Check sheet for the modelled part. Datum: model origin and axes. Units: mm. Face numbers are marked on the shaded views. Round coordinates to 2 decimals unless told otherwise and drop trailing zeros. Order: outer loops, then holes, each group sorted by start corner. A loop starts at its lowest first (then second) coordinate and runs counter-clockwise, first axis right, second up. Notation, with made-up numbers: (14.25, 16.5) -> (32.25, 16.5) arc R27 cw to (32.25, 49.5) -> close; hole circle Ø11 at (-30.5, 70). An arc over 180 degrees is marked (long way). Answer in a Markdown table with one row per item.
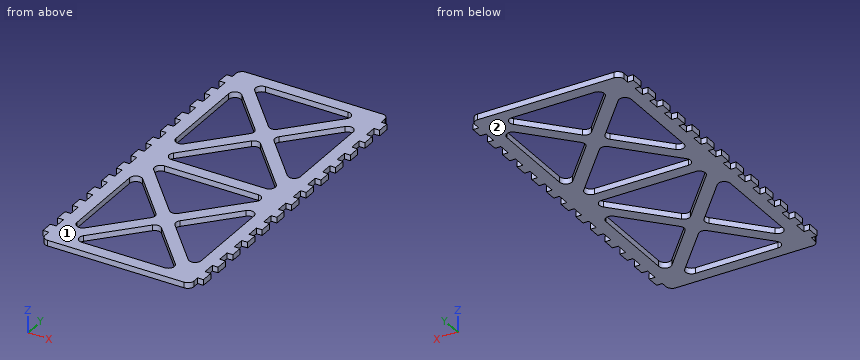
from build123d import *

# Parameters (mm, degrees)
SKETCH1_W                = 77.47
SKETCH1_H                = 171.45
BOSS_EXTRUDE1_DEPTH      = 1.4605
SKETCH3_W                = 2.921
SKETCH3_H                = 6.35
BOSS_EXTRUDE2_DEPTH      = 3
LPATTERN1_COUNT          = 13
LPATTERN1_PITCH          = 12.7
MIRROR1_COPY_1_SKETCH_W  = 2.921
MIRROR1_COPY_1_SKETCH_H  = 6.35
MIRROR1_COPY_1_DEPTH     = 3
MIRROR1_COPY_2_SKETCH_W  = 2.921
MIRROR1_COPY_2_SKETCH_H  = 6.35
MIRROR1_COPY_2_DEPTH     = 3
MIRROR1_COPY_3_SKETCH_W  = 2.921
MIRROR1_COPY_3_SKETCH_H  = 6.35
MIRROR1_COPY_3_DEPTH     = 3
MIRROR1_COPY_4_SKETCH_W  = 2.921
MIRROR1_COPY_4_SKETCH_H  = 6.35
MIRROR1_COPY_4_DEPTH     = 3
MIRROR1_COPY_5_SKETCH_W  = 2.921
MIRROR1_COPY_5_SKETCH_H  = 6.35
MIRROR1_COPY_5_DEPTH     = 3
MIRROR1_COPY_6_SKETCH_W  = 2.921
MIRROR1_COPY_6_SKETCH_H  = 6.35
MIRROR1_COPY_6_DEPTH     = 3
MIRROR1_COPY_7_SKETCH_W  = 2.921
MIRROR1_COPY_7_SKETCH_H  = 6.35
MIRROR1_COPY_7_DEPTH     = 3
MIRROR1_COPY_8_SKETCH_W  = 2.921
MIRROR1_COPY_8_SKETCH_H  = 6.35
MIRROR1_COPY_8_DEPTH     = 3
MIRROR1_COPY_9_SKETCH_W  = 2.921
MIRROR1_COPY_9_SKETCH_H  = 6.35
MIRROR1_COPY_9_DEPTH     = 3
MIRROR1_COPY_10_SKETCH_W = 2.921
MIRROR1_COPY_10_SKETCH_H = 6.35
MIRROR1_COPY_10_DEPTH    = 3
MIRROR1_COPY_11_SKETCH_W = 2.921
MIRROR1_COPY_11_SKETCH_H = 6.35
MIRROR1_COPY_11_DEPTH    = 3
MIRROR1_COPY_12_SKETCH_W = 2.921
MIRROR1_COPY_12_SKETCH_H = 6.35
MIRROR1_COPY_12_DEPTH    = 3
CUT_EXTRUDE1_DEPTH       = 96.389297571
FILLET1_R                = 3.175
FILLET2_R                = 3.175


with BuildPart() as part:
    # Sketch1 → Boss-Extrude1 (new, symmetric)
    with BuildSketch(Plane.XY):
        Rectangle(SKETCH1_W, SKETCH1_H)
    extrude(amount=BOSS_EXTRUDE1_DEPTH, both=True)

    # Sketch3 → Boss-Extrude2 (add)
    with BuildSketch(Plane.ZY.offset(38.735)):
        with Locations((0, -76.2)):
            Rectangle(SKETCH3_W, SKETCH3_H)
    boss_extrude2 = extrude(amount=BOSS_EXTRUDE2_DEPTH)

    # LPattern1: Boss-Extrude2 ×13
    with Locations(*[(0, i * LPATTERN1_PITCH, 0) for i in range(1, LPATTERN1_COUNT)]):
        add(boss_extrude2)

    # Mirror1: Boss-Extrude2 across plane
    add(boss_extrude2.mirror(Plane.ZY))

    # Mirror1 copy 1 sketch → Mirror1 copy 1 (add)
    with BuildSketch(Plane(origin=(38.735, 12.7, 0), x_dir=(0, 0, 1), z_dir=(1, 0, 0))):
        with Locations((0, 76.2)):
            Rectangle(MIRROR1_COPY_1_SKETCH_W, MIRROR1_COPY_1_SKETCH_H)
    extrude(amount=MIRROR1_COPY_1_DEPTH)

    # Mirror1 copy 2 sketch → Mirror1 copy 2 (add)
    with BuildSketch(Plane(origin=(38.735, 25.4, 0), x_dir=(0, 0, 1), z_dir=(1, 0, 0))):
        with Locations((0, 76.2)):
            Rectangle(MIRROR1_COPY_2_SKETCH_W, MIRROR1_COPY_2_SKETCH_H)
    extrude(amount=MIRROR1_COPY_2_DEPTH)

    # Mirror1 copy 3 sketch → Mirror1 copy 3 (add)
    with BuildSketch(Plane(origin=(38.735, 38.1, 0), x_dir=(0, 0, 1), z_dir=(1, 0, 0))):
        with Locations((0, 76.2)):
            Rectangle(MIRROR1_COPY_3_SKETCH_W, MIRROR1_COPY_3_SKETCH_H)
    extrude(amount=MIRROR1_COPY_3_DEPTH)

    # Mirror1 copy 4 sketch → Mirror1 copy 4 (add)
    with BuildSketch(Plane(origin=(38.735, 50.8, 0), x_dir=(0, 0, 1), z_dir=(1, 0, 0))):
        with Locations((0, 76.2)):
            Rectangle(MIRROR1_COPY_4_SKETCH_W, MIRROR1_COPY_4_SKETCH_H)
    extrude(amount=MIRROR1_COPY_4_DEPTH)

    # Mirror1 copy 5 sketch → Mirror1 copy 5 (add)
    with BuildSketch(Plane(origin=(38.735, 63.5, 0), x_dir=(0, 0, 1), z_dir=(1, 0, 0))):
        with Locations((0, 76.2)):
            Rectangle(MIRROR1_COPY_5_SKETCH_W, MIRROR1_COPY_5_SKETCH_H)
    extrude(amount=MIRROR1_COPY_5_DEPTH)

    # Mirror1 copy 6 sketch → Mirror1 copy 6 (add)
    with BuildSketch(Plane(origin=(38.735, 76.2, 0), x_dir=(0, 0, 1), z_dir=(1, 0, 0))):
        with Locations((0, 76.2)):
            Rectangle(MIRROR1_COPY_6_SKETCH_W, MIRROR1_COPY_6_SKETCH_H)
    extrude(amount=MIRROR1_COPY_6_DEPTH)

    # Mirror1 copy 7 sketch → Mirror1 copy 7 (add)
    with BuildSketch(Plane(origin=(38.735, 88.9, 0), x_dir=(0, 0, 1), z_dir=(1, 0, 0))):
        with Locations((0, 76.2)):
            Rectangle(MIRROR1_COPY_7_SKETCH_W, MIRROR1_COPY_7_SKETCH_H)
    extrude(amount=MIRROR1_COPY_7_DEPTH)

    # Mirror1 copy 8 sketch → Mirror1 copy 8 (add)
    with BuildSketch(Plane(origin=(38.735, 101.6, 0), x_dir=(0, 0, 1), z_dir=(1, 0, 0))):
        with Locations((0, 76.2)):
            Rectangle(MIRROR1_COPY_8_SKETCH_W, MIRROR1_COPY_8_SKETCH_H)
    extrude(amount=MIRROR1_COPY_8_DEPTH)

    # Mirror1 copy 9 sketch → Mirror1 copy 9 (add)
    with BuildSketch(Plane(origin=(38.735, 114.3, 0), x_dir=(0, 0, 1), z_dir=(1, 0, 0))):
        with Locations((0, 76.2)):
            Rectangle(MIRROR1_COPY_9_SKETCH_W, MIRROR1_COPY_9_SKETCH_H)
    extrude(amount=MIRROR1_COPY_9_DEPTH)

    # Mirror1 copy 10 sketch → Mirror1 copy 10 (add)
    with BuildSketch(Plane(origin=(38.735, 127, 0), x_dir=(0, 0, 1), z_dir=(1, 0, 0))):
        with Locations((0, 76.2)):
            Rectangle(MIRROR1_COPY_10_SKETCH_W, MIRROR1_COPY_10_SKETCH_H)
    extrude(amount=MIRROR1_COPY_10_DEPTH)

    # Mirror1 copy 11 sketch → Mirror1 copy 11 (add)
    with BuildSketch(Plane(origin=(38.735, 139.7, 0), x_dir=(0, 0, 1), z_dir=(1, 0, 0))):
        with Locations((0, 76.2)):
            Rectangle(MIRROR1_COPY_11_SKETCH_W, MIRROR1_COPY_11_SKETCH_H)
    extrude(amount=MIRROR1_COPY_11_DEPTH)

    # Mirror1 copy 12 sketch → Mirror1 copy 12 (add)
    with BuildSketch(Plane(origin=(38.735, 152.4, 0), x_dir=(0, 0, 1), z_dir=(1, 0, 0))):
        with Locations((0, 76.2)):
            Rectangle(MIRROR1_COPY_12_SKETCH_W, MIRROR1_COPY_12_SKETCH_H)
    extrude(amount=MIRROR1_COPY_12_DEPTH)

    # Sketch4 → Cut-Extrude1 (cut, through all)
    with BuildSketch(Plane.XY.offset(1.4605)):
        Polygon((0, 47.597902846), (28.717080391, 79.375), (-28.717080391, 79.375), align=None)
        Polygon((-32.385, 11.762042191), (-4.279401091, 42.8625), (-32.385, 73.962957809), align=None)
        Polygon((32.385, 73.962957809), (4.279401091, 42.8625), (32.385, 11.762042191), align=None)
        Polygon((31.58633965, 3.175), (0, 38.127097154), (-31.58633965, 3.175), align=None)
        Polygon((-31.58633965, -3.175), (0, -38.127097154), (31.58633965, -3.175), align=None)
        Polygon((-4.279401091, -42.8625), (-32.385, -11.762042191), (-32.385, -73.962957809), align=None)
        Polygon((28.717080391, -79.375), (0, -47.597902846), (-28.717080391, -79.375), align=None)
        Polygon((32.385, -73.962957809), (32.385, -11.762042191), (4.279401091, -42.8625), align=None)
    extrude(amount=-CUT_EXTRUDE1_DEPTH, mode=Mode.SUBTRACT)

    # Fillet1
    fillet1_edges = [part.edges().sort_by_distance(p)[0] for p in [
        (-31.58633965, -3.175, 0),
        (31.58633965, -3.175, 0),
        (0, -38.127097154, 0),
        (-31.58633965, 3.175, 0),
        (0, 38.127097154, 0),
        (31.58633965, 3.175, 0),
        (32.385, 73.962957809, 0),
        (32.385, 11.762042191, 0),
        (4.279401091, 42.8625, 0),
        (-32.385, 73.962957809, 0),
        (-4.279401091, 42.8625, 0),
        (-32.385, 11.762042191, 0),
        (32.385, -11.762042191, 0),
        (32.385, -73.962957809, 0),
        (4.279401091, -42.8625, 0),
        (-32.385, -11.762042191, 0),
        (-4.279401091, -42.8625, 0),
        (-32.385, -73.962957809, 0),
        (-28.717080391, -79.375, 0),
        (0, -47.597902846, 0),
        (28.717080391, -79.375, 0),
        (-28.717080391, 79.375, 0),
        (28.717080391, 79.375, 0),
        (0, 47.597902846, 0),
    ]]
    fillet(fillet1_edges, radius=FILLET1_R)

    # Fillet2
    fillet2_edges = [part.edges().sort_by_distance(p)[0] for p in [
        (-38.735, 85.725, 0),
        (38.735, 85.725, 0),
        (38.735, -85.725, 0),
        (-38.735, -85.725, 0),
    ]]
    fillet(fillet2_edges, radius=FILLET2_R)


solid = part.part
Item 1: Cross-section at D-D (z = 0.85). State how many separate pieces and enclosed holes the cut face has, and give its area (3 significant figures).
Result sheet:
| item | result |
|---|---|
| separate pieces | 1 |
| enclosed holes | 8 |
| area | 6,460 mm^2 |
Item 2: Cross-section at A-A (y = 13.5). Record the boundary of the cut face in (x, z) (1 decimal), and give its area (3 significant figures).
Result sheet:
| item | result |
|---|---|
| outline | (-41.7, -1.5) -> (-22.3, -1.5) -> (-22.3, 1.5) -> (-41.7, 1.5) -> close; (22.3, -1.5) -> (41.7, -1.5) -> (41.7, 1.5) -> (22.3, 1.5) -> close |
| area | 114 mm^2 |
Item 3: Depth check by flat-ended pin: P1, Ø0.9, axis at x = -40.5, z = 0, coming from the -Y side (3 decimals). Enter the tip coordinate at first touch or a pass-through.
Result sheet:
| item | result |
|---|---|
| P1 | stops at y = -79.375 |
Item 4: Scan lines: line 1 (X direction, y = -42.5, z = 0.8) (3 decimals); line 2 (Y direction, x = -25.5, z = 1.2) (3 decimals); line 3 (Y direction, x = -26, z = -0.35) (3 decimals). Record each from-to range of solid material in increasing order. Write a range as [from, to].
Result sheet:
| item | result |
|---|---|
| line 1 | x = [-38.735, -32.385], [-5.405, 5.405], [32.385, 38.735] |
| line 2 | y = [-85.725, -66.344], [-19.381, -9.91], [-3.358, 3.358], [9.91, 19.381], [66.344, 85.725] |
| line 3 | y = [-85.725, -66.898], [-18.827, -9.357], [-3.586, 3.586], [9.357, 18.827], [66.898, 85.725] |
Item 5: Cross-section at C-C (y = -24). Record the boundary of the cut face in (x, z) (1 decimal), and give its area (3 significant figures).
Result sheet:
| item | result |
|---|---|
| outline | (-41.7, -1.5) -> (-32.4, -1.5) -> (-32.4, 1.5) -> (-41.7, 1.5) -> close; (-21.3, -1.5) -> (-12.8, -1.5) -> (-12.8, 1.5) -> (-21.3, 1.5) -> close; (12.8, -1.5) -> (21.3, -1.5) -> (21.3, 1.5) -> (12.8, 1.5) -> close; (32.4, -1.5) -> (41.7, -1.5) -> (41.7, 1.5) -> (32.4, 1.5) -> close |
| area | 105 mm^2 |
Item 6: Mould release check, pull along Z, two halves, no side actions. Record for the marked faces 1 and 2: pulls with the +Z half, pulls with the -Z half, needs draft (parallel to the pull), parting line crosses it, or undercut.
Result sheet:
| item | result |
|---|---|
| face 1 | pulls with the +Z half |
| face 2 | pulls with the -Z half |
Item 7: Cross-section at B-B (x = -11). Record the boundary of the cut face in (y, z) (1 decimal), and give its area (3 significant figures).
Result sheet:
| item | result |
|---|---|
| outline | (-85.7, -1.5) -> (-79.4, -1.5) -> (-79.4, 1.5) -> (-85.7, 1.5) -> close; (-59.8, -1.5) -> (-50.3, -1.5) -> (-50.3, 1.5) -> (-59.8, 1.5) -> close; (-35.4, -1.5) -> (-26, -1.5) -> (-26, 1.5) -> (-35.4, 1.5) -> close; (-3.2, -1.5) -> (3.2, -1.5) -> (3.2, 1.5) -> (-3.2, 1.5) -> close; (26, -1.5) -> (35.4, -1.5) -> (35.4, 1.5) -> (26, 1.5) -> close; (50.3, -1.5) -> (59.8, -1.5) -> (59.8, 1.5) -> (50.3, 1.5) -> close; (79.4, -1.5) -> (85.7, -1.5) -> (85.7, 1.5) -> (79.4, 1.5) -> close |
| area | 166 mm^2 |
